Source: three-view drawing plus pictorial views. Frame: mm from the lowest corner of the part. A direction names the side the tool comes from. Coordinates: 2 decimals unless noted, no trailing zeros. Return JSON: item names as keys, results as strings.
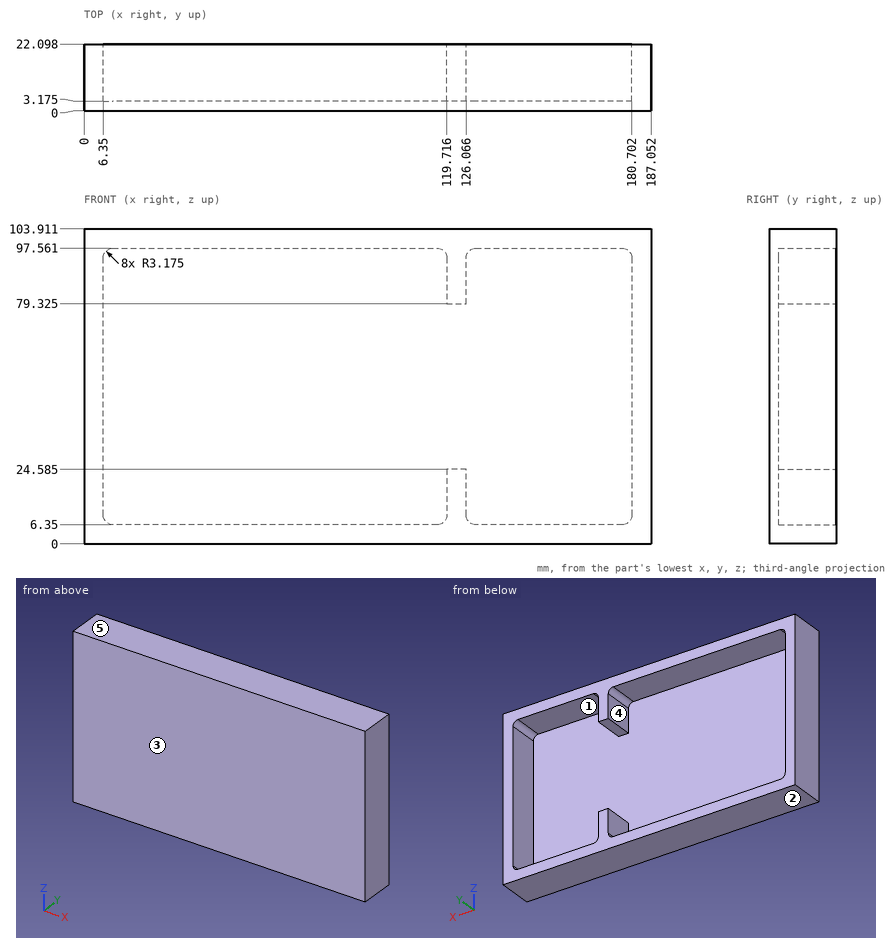
Item 1: First-contact query: pin 1 Ø8 at (x, z) = (55, 92) entering from +Y (1 decimal). Flat tip, straight axial feed; report the tip coordinate or a pass-through.
Worked out:
{"pin 1": "y = 3.2"}
Item 2: Mould query, pull axis Z, two halves, no side actions, for the marked faces 1, 2 and 3. Classes: +Z half, -Z half, draft (parallel to the pull), parting line (faces both ways), or undercut.
Worked out:
{"face 1": "undercut", "face 2": "-Z half", "face 3": "draft"}
Item 3: Ray query, probe 1 along X at (y, z) = (14.5, 87.5); probe 2 along X at (y, z) = (17.5, 37.5); probe 3 along Z at (x, y) = (131, 13). Return the intervals inside material, ascending. Write a range as from..to.
Worked out:
{"probe 1": "0..6.35, 119.72..126.07, 180.7..187.05", "probe 2": "0..6.35, 180.7..187.05", "probe 3": "0..6.35, 97.56..103.91"}
Item 4: Reachability of the marked faces 4 and 5 from +Z, -Z, +X, -X, +Y, -Y: full face, straight path, thin tool, end or side. Return the list, or none.
Worked out:
{"face 4": "+Y", "face 5": "+Z, +X, -X, +Y, -Y"}
